from build123d import *

# Parameters (mm, degrees)
SKETCH1_W           = 163.150096709
SKETCH1_H           = 382
BOSS_EXTRUDE1_DEPTH = 2
SKETCH2_W           = 86.892857143
SKETCH2_H           = 128
CUT_EXTRUDE1_DEPTH  = 582.357037259
SKETCH3_W           = 86.892857143
SKETCH3_H           = 100
CUT_EXTRUDE2_DEPTH  = 582.357037259
DRAFT1_ANGLE        = -31.857998891
DRAFT2_ANGLE        = 31.857998891
CUT_EXTRUDE3_DEPTH  = 581.711321285
FILLET1_R           = 5


with BuildPart() as part:
    # Sketch1 → Boss-Extrude1 (new body)
    with BuildSketch(Plane(origin=(184.061246273, -296.190511244, 0), x_dir=(-0.8493588352433418, -0.5278158476155048, 0), z_dir=(-0.5278158476155048, 0.8493588352433418, 0))):
        with Locations((-337.492534105, -211)):
            Rectangle(SKETCH1_W, SKETCH1_H)
    extrude(amount=-BOSS_EXTRUDE1_DEPTH)

    # Sketch2 → Cut-Extrude1 (cut, through all)
    with BuildSketch(Plane(origin=(185.116877969, -297.889228915, 0), x_dir=(0.8493588352433415, 0.5278158476155054, 0), z_dir=(0.5278158476155053, -0.8493588352433414, 0))):
        with Locations((299.363914323, -56)):
            Rectangle(SKETCH2_W, SKETCH2_H)
    extrude(amount=-CUT_EXTRUDE1_DEPTH, mode=Mode.SUBTRACT)

    # Sketch3 → Cut-Extrude2 (cut, through all)
    with BuildSketch(Plane(origin=(185.116877969, -297.889228915, 0), x_dir=(0.8493588352433415, 0.5278158476155054, 0), z_dir=(0.5278158476155053, -0.8493588352433414, 0))):
        with Locations((299.363914323, -352)):
            Rectangle(SKETCH3_W, SKETCH3_H)
    extrude(amount=-CUT_EXTRUDE2_DEPTH, mode=Mode.SUBTRACT)

    # Draft1
    draft1_faces = [part.faces().sort_by_distance(p)[0] for p in [
        (540.527815848, -75.849358835, -211),
    ]]
    draft(draft1_faces, Plane(origin=(184.061246273, -296.190511244, 0), x_dir=(0.8493588352433418, 0.5278158476155048, 0), z_dir=(-0.5278158476155048, 0.8493588352433418, 0)), DRAFT1_ANGLE)

    # Draft2
    draft2_faces = [part.faces().sort_by_distance(p)[0] for p in [
        (401.954839737, -161.962565418, -211),
    ]]
    draft(draft2_faces, Plane(origin=(184.061246273, -296.190511244, 0), x_dir=(0.8493588352433418, 0.5278158476155048, 0), z_dir=(-0.5278158476155048, 0.8493588352433418, 0)), DRAFT2_ANGLE)

    # Sketch4 → Cut-Extrude3 (cut, through all)
    with BuildSketch(Plane(origin=(185.116877969, -297.889228915, 0), x_dir=(0.8493588352433418, 0.5278158476155048, 0), z_dir=(0.5278158476155048, -0.8493588352433418, 0))):
        with BuildLine():
            Line((342.810342894, -20), (364.810342894, -20))
            add(Edge.make_bspline(
                [(342.810342894, -42), (346.302683554, -39.942808378), (351.300668251, -36.660712559), (356.350274178, -31.060781412), (361.089343651, -26.696748792), (363.56593564, -22.694365369), (364.810342894, -20)],
                knots=[0, 0, 0, 0, 0.388085015, 0.560148038, 0.716552584, 1, 1, 1, 1], degree=3))
            Line((342.810342894, -42), (342.810342894, -20))
        make_face()
        with BuildLine():
            Line((342.810342894, -380), (342.810342894, -402))
            Line((342.810342894, -402), (364.810342894, -402))
            add(Edge.make_bspline(
                [(342.810342894, -380), (346.302683554, -382.057191622), (351.300668251, -385.339287441), (356.350274178, -390.939218588), (361.089343651, -395.303251208), (363.56593564, -399.305634631), (364.810342894, -402)],
                knots=[0, 0, 0, 0, 0.388085015, 0.560148038, 0.716552584, 1, 1, 1, 1], degree=3))
        make_face()
    extrude(amount=-CUT_EXTRUDE3_DEPTH, mode=Mode.SUBTRACT)

    # Fillet1
    fillet1_edges = [part.edges().sort_by_distance(p)[0] for p in [
        (494.443950046, -104.487189726, -20),
        (475.758055671, -116.099138374, -42),
        (494.443950046, -104.487189726, -402),
        (475.758055671, -116.099138374, -380),
    ]]
    fillet(fillet1_edges, radius=FILLET1_R)


solid = part.part
CAD build for the part. Positions are in the model's coordinates, mm. Coordinates: 2 decimals unless noted, no trailing zeros. Write each loop counter-clockwise with the first axis right and the second up, starting at its lowest first coordinate (ties: lowest second). Pieces come first, ordered by that corner, then holes. Notation, with made-up numbers: M 28.25,37 L 56.25,37 A24 cw 56.25,71 Z; hole C 5.25,-33 d8. An arc over 180 degrees is marked long. Answer as a JSON object with one key per item and string values. Group by question number.
1) Saw through at B-B (y = -81.5). Write the cut outline in (x, z).
2) Saw through at A-A (z = -102). Write the cut outline in (x, y), plus the area to 3 significant figures.
3) Wall check: line 1 (Y direction, x = 514.5, z = -125); line 2 (Y direction, x = 409, z = -167.5); line 3 (X direction, y = -116, z = -303). Give the ranges that are in metal, low to high. Write a range as from..to.
4) Pin check, flat tips, straight feed: pin 1 Ø1 at (x, z) = (513.5, -295) entering from +Y; pin 2 Ø4 at (y, z) = (-126.5, -280) entering from +X; pin 3 Ø2 at (y, z) = (-122.5, -241.5) entering from -X. Stop position of each tip, or through.
Values follow:
{
 "1": {"outline": "M 529.54,-402 L 533.33,-402 L 533.33,-20 L 529.54,-20 Z"},
 "2": {"outline": "M 475.23,-115.25 L 476.29,-116.95 L 540,-77.35 L 540,-75 Z", "area": "151 mm2"},
 "3": {"line 1": "y = -93.2..-90.85", "line 2": "y = -158.76..-156.41", "line 3": "x = 475.7..477.81"},
 "4": {"pin 1": "stops at y = -91.16", "pin 2": "stops at x = 464.13", "pin 3": "stops at x = 461.95"}
}
